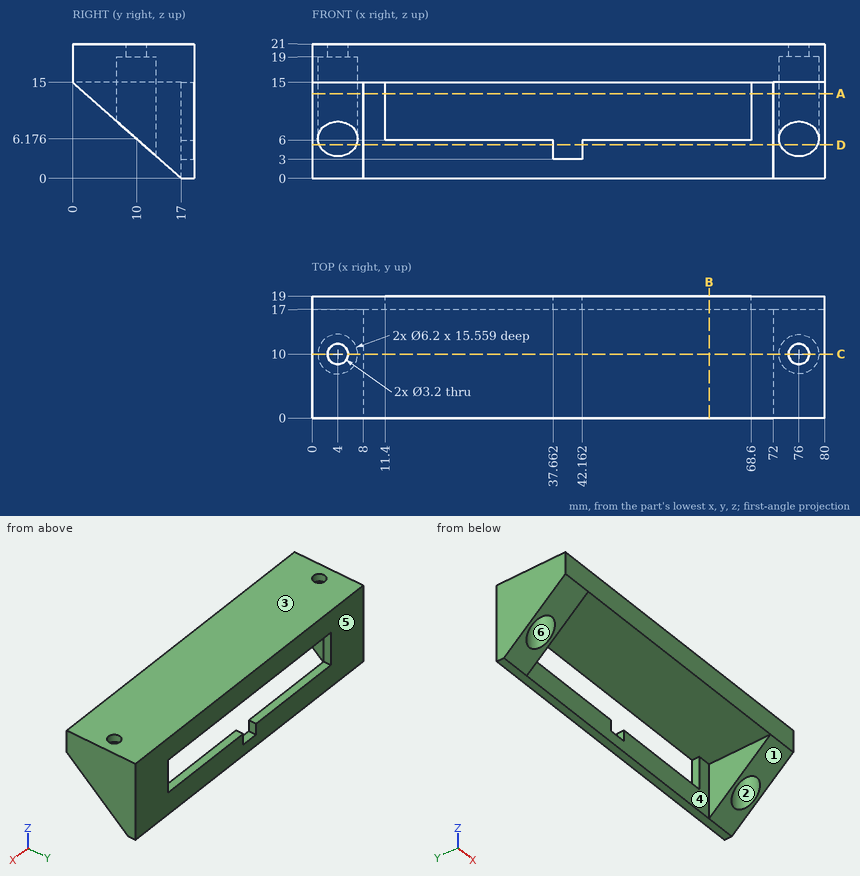
Part print with two shaded views. Sizes in mm from the minimum x, y, z corner. A direction names the side the tool comes from. Coordinates: 2 decimals unless noted, no trailing zeros. Write each loop counter-clockwise with the first axis right and the second up, starting at its lowest first coordinate (ties: lowest second). Pieces come first, ordered by that corner, then holes.
1. Drill centre lines: probe 1 along X at (y, z) = (10, 19.7); probe 2 along X at (y, z) = (10, 7.5); probe 3 along X at (y, z) = (6, 10.5). Where is each one in solid material? Low to high.
Answer block:
probe 1: x = 0 to 2.4, 5.6 to 74.4, 77.6 to 80
probe 2: x = 0 to 0.9, 7.1 to 8, 72 to 72.9, 79.1 to 80
probe 3: x = 0 to 8, 72 to 80
2. Band-saw the part on D-D, the plane z = 5.25. Give the cut face in (x, y), and give its area (3 significant figures).
Answer block:
outline: (0, 11.05) - (1.08, 11.05) arc R3.1 cw to (6.92, 11.05) - (8, 11.05) - (8, 17) - (37.66, 17) - (37.66, 19) - (0, 19) - close; (42.16, 17) - (72, 17) - (72, 11.05) - (73.08, 11.05) arc R3.1 cw to (78.92, 11.05) - (80, 11.05) - (80, 19) - (42.16, 19) - close
area: 229 mm2
3. Pull direction Z, two halves, no side cores. Call the marked faces 1, 2 and 3: released by +Z, released by -Z, zero draft, split by the parting line, or undercut.
Answer block:
face 1: released by -Z
face 2: zero draft
face 3: released by +Z
4. 3-axis set-ups, long thin cutter, end or side, ignore diameter. For the marked faces 4, 5 and 6: which of +Z, -Z, +X, -X, +Y, -Y reach the whole face in a straight line?
Answer block:
face 4: -Z, -Y
face 5: +Z, -Z, +X, -X, +Y
face 6: -Z
5. Band-saw the part on B-B, the plane x = 62. Give the cut face in (y, z).
Answer block:
outline: (0, 15) - (19, 15) - (19, 21) - (0, 21) - close; (17, 0) - (19, 0) - (19, 6) - (17, 6) - close
6. Band-saw the part on C-C, the plane y = 10. Give the cut face in (x, z).
Answer block:
outline: (0, 6.18) - (0.9, 6.18) - (0.9, 19) - (2.4, 19) - (2.4, 21) - (0, 21) - close; (5.6, 19) - (7.1, 19) - (7.1, 6.18) - (8, 6.18) - (8, 15) - (72, 15) - (72, 6.18) - (72.9, 6.18) - (72.9, 19) - (74.4, 19) - (74.4, 21) - (5.6, 21) - close; (77.6, 19) - (79.1, 19) - (79.1, 6.18) - (80, 6.18) - (80, 21) - (77.6, 21) - close
7. Drop flat-ended pins along their axis: pin 1 (3 mm diameter, centred on x = 60.5, z = 12, fed in from -Y); pin 2 (1 mm diameter, centred on x = 45.5, y = 14, fed in from -Z); pin 3 (12 mm diameter, centred on x = 56, z = 8, fed in from -Y); pin 4 (8 mm diameter, centred on x = 4, y = 10, fed in from -Z). Give the stop position or say it passes through.
Answer block:
pin 1: passes through
pin 2: stops at z = 15
pin 3: stops at y = 17
pin 4: stops at z = 2.65
8. Band-saw the part on A-A, the plane z = 13.25. Give the cut face in (x, y).
Answer block:
outline: (0, 1.98) - (8, 1.98) - (8, 17) - (11.4, 17) - (11.4, 19) - (0, 19) - close; (68.6, 17) - (72, 17) - (72, 1.98) - (80, 1.98) - (80, 19) - (68.6, 19) - close; hole circle Ø6.2 at (4, 10); hole circle Ø6.2 at (76, 10)
